Source: three-view drawing plus pictorial views. Frame: mm from the lowest corner of the part. Coordinates: 2 decimals unless noted, no trailing zeros. Write each loop counter-clockwise with the first axis right and the second up, starting at its lowest first coordinate (ties: lowest second). Pieces come first, ordered by that corner, then holes. Notation, with made-up numbers: (-33.75, -31.75) -> (25.25, -31.75) arc R10 ccw to (25.25, -13.75) -> close; hole circle Ø6 at (23, 20). An arc over 180 degrees is marked (long way). One line per item, written item: value.
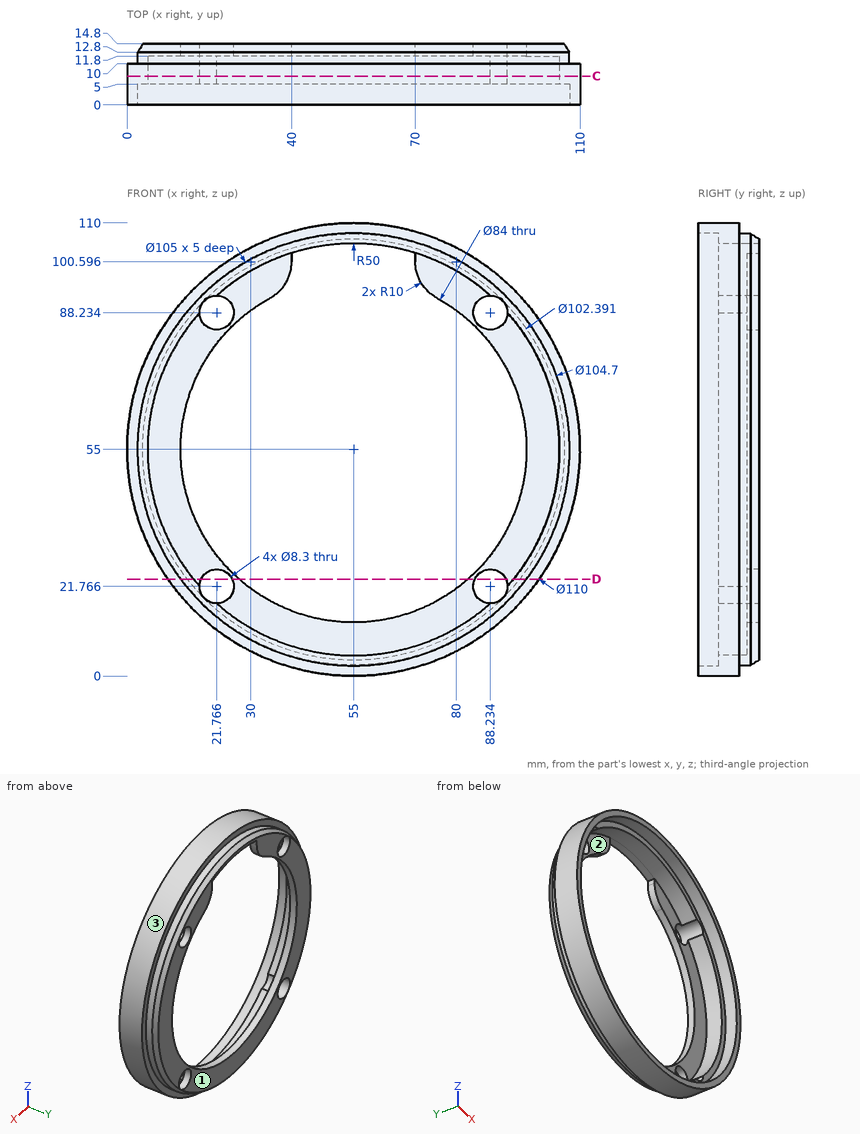
(1) Section C-C (y = 7). Return the cut outline in (x, z), then the cut area to 3 significant figures.
Responses:
outline: circle Ø110 at (55, 55); hole (17.62, 21.8) arc R4.15 ccw to (21.8, 17.62) arc R50 ccw to (88.2, 17.62) arc R4.15 ccw to (92.38, 21.8) arc R50 ccw to (92.38, 88.2) arc R4.15 ccw to (88.2, 92.38) arc R50 ccw to (21.8, 92.38) arc R4.15 ccw to (17.62, 88.2) arc R50 ccw to start
area: 1,630 mm2
(2) First-contact query: pin 1 (3 mm diameter, centred on x = 52.5, y = 2.5, fed in from -Z); pin 2 (6 mm diameter, centred on y = 13.5, z = 74.5, fed in from +X); pin 3 (6 mm diameter, centred on y = 10, z = 91, fed in from +X); pin 4 (7.5 mm diameter, centred on x = 21.77, z = 88.23, fed in from +Y). Flat tips, straight axial feed; report the tip coordinate or a pass-through.
Responses:
pin 1: stops at z = 0.01
pin 2: stops at x = 104.65
pin 3: stops at x = 99
pin 4: passes through
(3) Line query: line 1 (X direction, y = 2.2, z = 55); line 2 (X direction, y = 14, z = 86.5) (1 decimal); line 3 (X direction, y = 12.8, z = 55). Output: solid intervals per line, ascending. Write a range as [from, to].
Responses:
line 1: x = [0, 2.5], [107.5, 110]
line 2: x = [14.1, 18], [25.5, 27.2], [82.8, 84.5], [92, 95.9]
line 3: x = [2.65, 13], [97, 107.35]
(4) Pull-direction query (Z, two-part tool) for the marked faces 1, 2 and 3; classes: released by +Z, released by -Z, zero draft, split by the parting line, or undercut.
Responses:
face 1: zero draft
face 2: undercut
face 3: split by the parting line
(5) Section D-D (z = 23.5). State how many separate pieces and enclosed holes the cut face has, then the cut area to 3 significant figures.
Responses:
separate pieces: 4
enclosed holes: 0
area: 140 mm2
